Could you check a few things on this model? Use its own coordinates, in mm. A direction names the side the tool comes from. Coordinates: 2 decimals unless noted, no trailing zeros. Write each loop counter-clockwise with the first axis right and the second up, starting at its lowest first coordinate (ties: lowest second). Pieces come first, ordered by that corner, then holes. Notation, with made-up numbers: M -4,-9.5 L 47,-9.5 A23 ccw 47,21.5 Z; hole C 46.5,-18.5 d7. An arc over 180 degrees is marked long. Write item = value, one per line.
```python
from build123d import *

# Parameters (mm, degrees)
F2_R     = 2
F3_SIZE2 = 1.8198511713
F3_SIZE  = 5
F4_R     = 2
F5_D     = 3
F5_DEPTH = 10.0010001


with BuildPart() as f1:
    # F0 (on Front) → F1 (revolve)
    with BuildSketch(Plane.XZ):
        Polygon((-50, 0), (0, 0), (0, 10), (-3, 10), (-3, 6), (-50, 6), align=None)
    revolve(axis=Axis((-25, 0, 0), (1, 0, 0)))

    # F2
    f2_edges = [f1.edges().sort_by_distance(p)[0] for p in [
        (0, 0, -10),
    ]]
    fillet(f2_edges, radius=F2_R)

    # F3
    f3_edges = [f1.edges().sort_by_distance(p)[0] for p in [
        (-50, 0, -6),
    ]]
    chamfer(f3_edges, length=F3_SIZE, length2=F3_SIZE2)

    # F4
    f4_edges = [f1.edges().sort_by_distance(p)[0] for p in [
        (-50, 0, -4.180149),
    ]]
    fillet(f4_edges, radius=F4_R)

    # F5 (through all, one way)
    with BuildSketch(Plane(origin=(0, 0, 0), x_dir=(1, 0, 0), z_dir=(0, 1, 0))):
        with Locations((-42.5, 0)):
            Circle(F5_D / 2)
    extrude(amount=-F5_DEPTH, mode=Mode.SUBTRACT)


solid = f1.part
```
Item 1: Imagine slicing it at B-B (x = -10). Write out the boundary of the cut face in (y, z).
Numbers:
outline = C 0,0 d12
Item 2: If I drill on line 1 along X through (y, z) = (-2, 0); line 2 along X through (y, z) = (-2, 7.5); line 3 along Z through (x, y) = (-42.5, -3.5), over which ranges is the centre line in solid material (lowest first)?
Numbers:
line_1 = -50 to -44, -41 to 0
line_2 = -3 to 0
line_3 = -4.87 to -1.5, 1.5 to 4.87
Item 3: For faces 1 (the face through (0, 0, 0)), 2 (the face through (-44, -3, 0)), 3 (the face through (-24.294, 5.857, -1.301)), which set-ups out of +Z, -Z, +X, -X, +Y, -Y let a thin tool reach every point of the face, with its end or its side?
Numbers:
face_1 = +Z, -Z, +X, +Y, -Y
face_2 = -Y
face_3 = -X
Item 4: Imagine slicing it at A-A (z = 0). Write out the boundary of the cut face in (x, y).
Numbers:
outline = M -50,-2.78 A2 ccw -48.68,-4.66 L -45,-6 L -44,-6 L -44,0 L -41,0 L -41,-6 L -3,-6 L -3,-10 L -2,-10 A2 ccw 0,-8 L 0,8 A2 ccw -2,10 L -3,10 L -3,6 L -45,6 L -48.68,4.66 A2 ccw -50,2.78 Z
Item 5: Imagine slicing it at C-C (x = -42). Write out the boundary of the cut face in (y, z), and give its area (3 significant figures).
Numbers:
outline = M -5.83,-1.41 A6 ccw long -5.83,1.41 L 0,1.41 L 0,-1.41 Z
area = 96.3 mm²
Item 6: I'm going to push flat-ended pins straight in: P1, Ø2, axis at x = -39, y = 3.5, coming from the +Z side; P2, Ø4, axis at x = -20, z = -2.5, coming from the +Y side; P3, Ø5, axis at x = -24.5, y = 3.5, coming from the -Z side. Where does each tip first touch, or does it pass through?
Numbers:
P1 = 5.45
P2 = 5.98
P3 = -5.92
Item 7: If we mould it in two halves opening along Z, with no side actions, what happens to faces 4 (the face through (-43, 0, 0)), 5 (the face through (-3, 0, 7)), 6 (the face through (-2.51, 9.76, -2.17))? For each: pulls with the +Z half, pulls with the -Z half, needs draft (parallel to the pull), parting line crosses it, or undercut.
Numbers:
face_4 = undercut
face_5 = needs draft
face_6 = parting line crosses it
